Input: part model. Units: mm. Frame: model coordinates. A direction names the side the tool comes from. Coordinates: 2 decimals unless noted, no trailing zeros. Order: outer loops, then holes, each group sorted by start corner. A loop starts at its lowest first (then second) coordinate and runs counter-clockwise, first axis right, second up. Notation, with made-up numbers: (-21, 65.25) -> (3, 65.25) arc R20 ccw to (3, 101.25) -> close; hole circle Ø2 at (46, 82). An arc over 180 degrees is marked (long way). One line per question, with ' | ' between items.
Autodesk Inventor part; units mm, degrees
ref_plane "YZ Plane" through (0, 0, 0) normal (1, 0, 0) x (0, 1, 0)
ref_plane "XZ Plane" through (0, 0, 0) normal (0, 1, 0) x (-1, 0, 0)
ref_plane "XY Plane" through (0, 0, 0) normal (0, 0, 1) x (1, 0, 0)
sketch "Sketch1" plane through (0, 0, 0) normal (0, 1, 0) x (-1, 0, 0)
  line L0 (0, 0) -> (150, 0)
  line L1 (150, 0) -> (150, -75)
  line L2 (150, -75) -> (0, -75)
  line L3 (0, -75) -> (0, 0)
  dimension "d0" = 150
  dimension "d1" = 75
extrude "Extrusion1" add sketch "Sketch1" along normal blind 6
sketch "Sketch6" plane through (-150, 0, 0) normal (0, 0, 1) x (1, 0, 0)
  line L0 (0, 6) -> (150, 6)
  line L1 (50, 82) -> (22.5, 6)
  line L2 (100, 82) -> (127.5, 6)
  line L3 (50, 82) -> (100, 82)
  line L4 (22.5, 6) -> (127.5, 6)
  line L5 (22.5, 6) -> (127.5, 6)
  line L6 (100, 82) -> (50, 82)
  line L7 (50, 82) -> (22.5, 6)
  line L8 (100, 82) -> (127.5, 6)
extrude "Extrusion2" add sketch "Sketch6" against normal blind 45
sketch "Sketch7" plane through (-150, 0, 0) normal (0, 0, 1) x (1, 0, 0)
  line L0 (150, 0) -> (0, 0)
  line L1 (75, 0) -> (75, 50)
  circle A0 centre (75, 50) radius 25
  dimension "d14" = 50
  dimension "d15" = 50
extrude "Extrusion3" add sketch "Sketch7" along normal blind 13
sketch "Sketch9" plane through (0, 0, 0) normal (1, 0, 0) x (0, 0, -1)
  line L0 (0, 6) -> (75, 6)
  line L1 (45, 82) -> (0, 82)
  line L2 (0, 82) -> (45, 82)
  line L3 (0, 6) -> (0, 9)
  line L4 (0, 6) -> (0, 82)
  line L5 (0, 9) -> (45, 9)
  line L6 (45, 6) -> (45, 82)
  line L7 (0, 82) -> (3, 82)
  line L8 (3, 82) -> (3, 9)
  line L9 (0, 82) -> (0, 79)
  line L10 (0, 79) -> (45, 79)
  line L11 (45, 79) -> (42, 79)
  line L12 (42, 79) -> (42, 6)
  line L13 (3, 9) -> (3, 79)
  line L14 (3, 79) -> (42, 79)
  line L15 (42, 79) -> (42, 9)
  line L16 (42, 9) -> (3, 9)
  dimension "d18" = 3
  dimension "d19" = 3
  dimension "d20" = 3
  dimension "d21" = 3
extrude "Extrusion4" cut sketch "Sketch9" against normal blind 150 contours L5 L8 L10 L12
sketch "Sketch10" plane through (-75, 50, 13) normal (0, 0, 1) x (1, 0, 0)
  circle A0 centre (0, 0) radius 25
  circle A1 centre (0, 0) radius 4.5
  point P0 (75, -50)
  dimension "d24" = 9
extrude "Extrusion5" cut sketch "Sketch10" against normal blind 150 contours A1
properties part number "Casing"
1. Cut plane B-B, the plane x = -75. Return loops of the section in (y, z).
Recorded:
outline: (0, -75) -> (6, -75) -> (6, -45) -> (45.5, -45) -> (45.5, -42) -> (9, -42) -> (9, -3) -> (45.5, -3) -> (45.5, 13) -> (25, 13) -> (25, 0) -> (0, 0) -> close; (54.5, -45) -> (82, -45) -> (82, 0) -> (75, 0) -> (75, 13) -> (54.5, 13) -> (54.5, -3) -> (79, -3) -> (79, -42) -> (54.5, -42) -> close
2. Cut plane C-C, the plane y = 20. Return loops of the section in (x, z), and give its area (3 significant figures).
Recorded:
outline: (-122.43, -45) -> (-27.57, -45) -> (-27.57, -42) -> (-122.43, -42) -> close; (-122.43, -3) -> (-27.57, -3) -> (-27.57, 0) -> (-122.43, 0) -> close | area: 569 mm^2
3. Mould query, pull axis X, two halves, no side actions, for faces 4 (the face through (-75.98, 45.61, -43.48)), 5 (the face through (-75, 79, -22)), 6 (the face through (-75.98, 45.61, 5.11)), 7 (the face through (-112.67, 46.99, -42.4)). Classes: released by +X, released by -X, zero draft, split by the parting line, or undercut.
Recorded:
face 4: undercut | face 5: zero draft | face 6: undercut | face 7: released by -X
4. Cut plane A-A, the plane z = -10.5. Return loops of the section in (x, y), and give its area (4 significant figures).
Recorded:
outline: (-150, 0) -> (0, 0) -> (0, 6) -> (-22.5, 6) -> (-23.59, 9) -> (-126.41, 9) -> (-127.5, 6) -> (-150, 6) -> close; (-101.09, 79) -> (-48.91, 79) -> (-50, 82) -> (-100, 82) -> close | area: 1,365 mm^2
5. Pin query (flat end, axial travel): pin 1 Ø12 at (y, z) = (72, -36.5) entering from -X; pin 2 Ø7 at (x, y) = (-75, 50) entering from -Z. Return the tip coordinate at first contact, or that it passes through.
Recorded:
pin 1: stops at x = -104.49 | pin 2: passes through
6. Cut plane D-D, the plane y = 50. Return loops of the section in (x, z), and give its area (3 significant figures).
Recorded:
outline: (-111.58, -45) -> (-79.5, -45) -> (-79.5, -42) -> (-111.58, -42) -> close; (-111.58, -3) -> (-79.5, -3) -> (-79.5, 13) -> (-100, 13) -> (-100, 0) -> (-111.58, 0) -> close; (-70.5, -45) -> (-38.42, -45) -> (-38.42, -42) -> (-70.5, -42) -> close; (-70.5, -3) -> (-38.42, -3) -> (-38.42, 0) -> (-50, 0) -> (-50, 13) -> (-70.5, 13) -> close | area: 918 mm^2
7. Access query for faces 1 (the face through (-76, 36, -45)), 2 (the face through (-95, 65, 6)), 3 (the face through (-74, 37, -3)). Directions: +Z, -Z, +X, -X, +Y, -Y. A direction counts if a zero-diameter tool reaches every point of the face in a straight line with its end or side. Return the directions, or none.
Recorded:
face 1: -Z, +X, -X, +Y | face 2: +Z | face 3: +X, -X
8. Ray query, line 1 (Z direction, x = -45.5, y = 66); line 2 (Y direction, x = -75, z = -43.75); line 3 (Y direction, x = -45, z = -20.5). Return the intervals inside material, ascending. Write a range as [from, to].
Recorded:
line 1: z = [-45, -42], [-3, 0] | line 2: y = [0, 45.5], [54.5, 82] | line 3: y = [0, 9]
